Can you work these out from the model? Positions are in its coordinate system, mm. A direction names the side the tool comes from. Give positions to 0.01 mm unless a question says otherwise; leave off trailing zeros. Order: outer loops, then holes, each group sorted by start corner. A loop starts at its lowest first (then second) coordinate and runs counter-clockwise, first axis right, second up. Notation, with made-up numbers: (-1.5, 19.5) - (9.5, 19.5) arc R11 ccw to (9.5, 28.5) - close; hole circle Ø4 at (-26, 89.5). An arc over 180 degrees is marked (long way). Answer as a JSON object with one key per item and string values.
```python
from build123d import *

# Parameters (mm, degrees)
BOSS_EXTRUDE1_DEPTH  = 3
SKETCH3_R            = 1.75
CUT_EXTRUDE2_DEPTH   = 4
LPATTERN1_COUNT      = 2
LPATTERN1_PITCH      = 70
LPATTERN1_COUNT_DIR2 = 2
LPATTERN1_PITCH_DIR2 = 90
SKETCH5_W            = 10
SKETCH5_H            = 10
CUT_EXTRUDE4_DEPTH   = 4


with BuildPart() as part:
    # Sketch1 → Boss-Extrude1 (new body)
    with BuildSketch(Plane(origin=(0, 0, 0), x_dir=(1, 0, 0), z_dir=(0, 1, 0))):
        with BuildLine():
            Line((-45, 40), (45, 40))
            ThreePointArc((45, 40), (48.535533906, 38.535533906), (50, 35))
            Line((50, 35), (50, -35))
            ThreePointArc((50, -35), (48.535533906, -38.535533906), (45, -40))
            Line((45, -40), (-45, -40))
            ThreePointArc((-45, -40), (-48.535533906, -38.535533906), (-50, -35))
            Line((-50, -35), (-50, 35))
            ThreePointArc((-50, 35), (-48.535533906, 38.535533906), (-45, 40))
        make_face()
    extrude(amount=BOSS_EXTRUDE1_DEPTH)

    # Sketch3 → Cut-Extrude2 (cut, through all)
    with BuildSketch(Plane(origin=(0, 3, 0), x_dir=(1, 0, 0), z_dir=(0, 1, 0))):
        with Locations((-45, -35)):
            Circle(SKETCH3_R)
    cut_extrude2 = extrude(amount=-CUT_EXTRUDE2_DEPTH, mode=Mode.SUBTRACT)

    # LPattern1: Cut-Extrude2 2 × 2
    with Locations(*[(j * LPATTERN1_PITCH_DIR2, 0, -i * LPATTERN1_PITCH) for i in range(LPATTERN1_COUNT) for j in range(LPATTERN1_COUNT_DIR2) if (i, j) != (0, 0)]):
        add(cut_extrude2, mode=Mode.SUBTRACT)

    # Sketch5 → Cut-Extrude4 (cut, through all)
    with BuildSketch(Plane(origin=(0, 3, 0), x_dir=(1, 0, 0), z_dir=(0, 1, 0))):
        with Locations((-35, 0)):
            Rectangle(SKETCH5_W, SKETCH5_H)
    extrude(amount=-CUT_EXTRUDE4_DEPTH, mode=Mode.SUBTRACT)


solid = part.part
```
Q1. I'm going to push a flat-ended pin straight in: pin 1 Ø2 at (x, z) = (45, -35) entering from -Y. Where does the tip first touch, or does it pass through?
Recorded:
{"pin 1": "passes through"}
Q2. We'd pull the mould along Z, two halves only. Please class faces 1 (the face through (46.617, 1.521, -34.33)), 2 (the face through (49, 1, 38)), 3 (the face through (-40, 2, 0)), 4 (the face through (1, 0, -1)): released by +Z, released by -Z, zero draft, split by the parting line, or undercut.
Recorded:
{"face 1": "undercut", "face 2": "released by +Z", "face 3": "undercut", "face 4": "zero draft"}
Q3. If we section it at A-A, the plane y = 2.45: Please give me the cut outline in (x, z).
Recorded:
{"outline": "(-50, -35) arc R5 ccw to (-45, -40) - (45, -40) arc R5 ccw to (50, -35) - (50, 35) arc R5 ccw to (45, 40) - (-45, 40) arc R5 ccw to (-50, 35) - close; hole circle Ø3.5 at (-45, -35); hole circle Ø3.5 at (-45, 35); hole (-40, -5) - (-30, -5) - (-30, 5) - (-40, 5) - close; hole circle Ø3.5 at (45, -35); hole circle Ø3.5 at (45, 35)"}
Q4. I need wall thicknesses on L1, parallel to X at y = 1.1, z = 35; L2, parallel to Z at x = -45, y = 1.3; L3, parallel to X at y = 2.55, z = -2. Which ranges of each line are inside material? Lowest first, please.
Recorded:
{"L1": "x = -50 to -46.75, -43.25 to 43.25, 46.75 to 50", "L2": "z = -40 to -36.75, -33.25 to 33.25, 36.75 to 40", "L3": "x = -50 to -40, -30 to 50"}
Q5. Which directions (+Z, -Z, +X, -X, +Y, -Y) give clear straight access to the entire face, cutting with the end or side of a thin tool? Please do faces 5 (the face through (-35, 2, -5)), 6 (the face through (-50, 1, 0)).
Recorded:
{"face 5": "+Y, -Y", "face 6": "+Z, -Z, -X, +Y, -Y"}
